Read the model definition and answer for the solid it produces. Units are mm, in the model's axes. A direction names the side the tool comes from. Coordinates: 2 decimals unless noted, no trailing zeros. Write each loop counter-clockwise with the first axis right and the second up, starting at its lowest first coordinate (ties: lowest second). Pieces come first, ordered by that corner, then holes. Notation, with made-up numbers: (-15.75, 18.25) - (-9.75, 18.25) arc R10 ccw to (-9.75, 30.25) - close; hole circle Ø5 at (23.5, 38). An arc over 180 degrees is marked (long way). Use a Markdown table: item, result.
Autodesk Inventor part; units mm, degrees
ref_plane "YZ Plane" through (0, 0, 0) normal (1, 0, 0) x (0, 1, 0)
ref_plane "XZ Plane" through (0, 0, 0) normal (0, 1, 0) x (-1, 0, 0)
ref_plane "XY Plane" through (0, 0, 0) normal (0, 0, 1) x (1, 0, 0)
sketch "Sketch1" plane through (0, 0, 0) normal (0, 1, 0) x (-1, 0, 0)
  line L0 (-40.135, 30.32) -> (40.135, 30.32)
  line L1 (40.135, 30.32) -> (40.135, -30.32)
  line L2 (40.135, -30.32) -> (-40.135, -30.32)
  line L3 (-40.135, -30.32) -> (-40.135, 30.32)
  line L4 (-40.135, 30.32) -> (40.135, -30.32) construction
  line L5 (40.135, 30.32) -> (-40.135, -30.32) construction
  point P0 (0, 0)
  dimension "d0" = 80.27
  dimension "d1" = 60.64
extrude "Extrusion1" add sketch "Sketch1" along normal blind 4.75
sketch "Sketch2" plane through (0, 4.75, 0) normal (0, 1, 0) x (1, 0, 0)
  line L0 (-40.135, -30.32) -> (40.135, -30.32)
  line L1 (40.135, -30.32) -> (40.135, 30.32)
  line L2 (-40.135, -30.32) -> (40.135, -30.32)
  line L3 (40.135, -30.32) -> (40.135, -25.57)
  line L4 (40.135, -25.57) -> (-40.135, -25.57)
  line L5 (-40.135, -25.57) -> (-40.135, -30.32)
  line L6 (-40.135, 30.32) -> (40.135, 30.32)
  line L7 (40.135, 30.32) -> (40.135, 25.57)
  line L8 (40.135, 25.57) -> (-40.135, 25.57)
  line L9 (-40.135, 25.57) -> (-40.135, 30.32)
  line L10 (-40.135, -25.57) -> (-35.385, -25.57)
  line L11 (-35.385, -25.57) -> (-35.385, 25.57)
  line L12 (-35.385, 25.57) -> (-40.135, 25.57)
  line L13 (-40.135, 25.57) -> (-40.135, -25.57)
  line L14 (40.135, 25.57) -> (35.385, 25.57)
  line L15 (35.385, 25.57) -> (35.385, -25.57)
  line L16 (35.385, -25.57) -> (40.135, -25.57)
  line L17 (40.135, -25.57) -> (40.135, 25.57)
  point P0 (0, 0)
  dimension "d4" = 4.75
  dimension "d5" = 4.75
  dimension "d6" = 4.75
  dimension "d7" = 4.75
extrude "Extrusion2" add sketch "Sketch2" along normal blind 50.72 contours L5 L4 L1 L0 | L13 L8 L11 L4 | L4 L15 L8 L1 | L9 L6 L1 L8
sketch "Sketch3" plane through (0, 55.47, 0) normal (0, 1, 0) x (1, 0, 0)
  line L0 (40.135, -30.32) -> (-40.135, -30.32)
  line L1 (-40.135, -30.32) -> (-40.135, 30.32)
  line L2 (-40.135, 30.32) -> (40.135, 30.32)
  line L3 (40.135, 30.32) -> (40.135, -30.32)
  point P0 (0, 0)
extrude "Extrusion3" add sketch "Sketch3" along normal blind 4.75
sketch "Sketch4" plane through (40.135, 0, 30.32) normal (1, 0, 0) x (0, 0, -1)
  line L0 (0, 60.22) -> (60.64, 60.22)
  line L1 (0, 0) -> (0, 60.22)
  line L2 (60.64, 0) -> (60.64, 60.22)
  line L3 (60.64, 0) -> (0, 0)
  point P0 (30.32, 0)
  point P1 (30.32, 30.11)
hole "Hole1" at (40.135, 30.11, 0) direction (-1, 0, 0) diameter 11.4554 end up to surface
sketch "Sketch5" plane through (0, 60.22, 0) normal (0, 1, 0) x (1, 0, 0)
  line L0 (-40.135, -30.32) -> (40.135, -30.32)
  line L1 (40.135, -30.32) -> (40.135, 30.32)
  line L2 (40.135, 30.32) -> (-40.135, 30.32)
  line L3 (-40.135, 30.32) -> (-40.135, -30.32)
  point P0 (0, 0)
  point P1 (-24.635, 0)
  point P2 (15.015, 0)
  dimension "d19" = 15.5
  dimension "d20" = 25.12
hole "Hole2" at (-24.635, 60.22, 0) at (15.015, 60.22, 0) direction (0, -1, 0) diameter 11.4554 end up to surface
properties part number "Reservoir" material "PMMA Plastic"
(1) For faces 1 (the cylindrical face through (-30.314, 57.812, -0.746)), 2 (the flat face through (0, 4.75, 0)), 3 (the cylindrical face through (37.73, 24.43, 0.75)), determine the directions among +Z, -Z, +X, -X, +Y, -Y from which every point of the face is accessible in a straight line to the end or side of a thin tool.
Report:
| item | result |
|---|---|
| face 1 | +Y |
| face 2 | none |
| face 3 | +X |
(2) Straight lines are drawn through the part: L1, parallel to X at y = 59.25, z = 0 (3 decimals); L2, parallel to X at y = 26, z = 11 (3 decimals); L3, parallel to Y at x = -0.5, z = 6.5. For each, find the intervals that lie inside material, in ascending order.
Report:
| item | result |
|---|---|
| L1 | x = -40.135 to -30.363, -18.907 to 9.287, 20.743 to 40.135 |
| L2 | x = -40.135 to -35.385, 35.385 to 40.135 |
| L3 | y = 0 to 4.75, 55.47 to 60.22 |
(3) The mould has two halves that part along Z. Classify faces 4 (the flat face through (-1, 30, -30.32)), 5 (the flat face through (35.385, 24, 0)), 6 (the flat face through (-40.135, 30, 0)): pulls with the +Z half, pulls with the -Z half, needs draft (parallel to the pull), parting line crosses it, or undercut.
Report:
| item | result |
|---|---|
| face 4 | pulls with the -Z half |
| face 5 | undercut |
| face 6 | needs draft |
(4) A cutting plane is placed at D-D, the plane y = 30.11. Write down the section's boundary in (x, z) (3 decimals), and give its area (3 significant figures).
Report:
| item | result |
|---|---|
| outline | (-40.135, -30.32) - (40.135, -30.32) - (40.135, -5.728) - (35.385, -5.728) - (35.385, -25.57) - (-35.385, -25.57) - (-35.385, 25.57) - (35.385, 25.57) - (35.385, 5.728) - (40.135, 5.728) - (40.135, 30.32) - (-40.135, 30.32) - close |
| area | 1,190 mm² |
(5) Each of these flat-tipped pins is pushed along its axis until it touches: P1, Ø7, axis at y = 30.11, z = 0, coming from the +X side (3 decimals); P2, Ø10.5, axis at x = -24.635, z = 0, coming from the +Y side. Where does it stop, or does it pass through?
Report:
| item | result |
|---|---|
| P1 | stops at x = -35.385 |
| P2 | stops at y = 4.75 |
(6) A cutting plane is placed at A-A, the plane y = 54. Write down the section's boundary in (x, z) (3 decimals), and give its area (3 significant figures).
Report:
| item | result |
|---|---|
| outline | (-40.135, -30.32) - (40.135, -30.32) - (40.135, 30.32) - (-40.135, 30.32) - close; hole (-35.385, -25.57) - (35.385, -25.57) - (35.385, 25.57) - (-35.385, 25.57) - close |
| area | 1,250 mm² |
(7) A cutting plane is placed at B-B, the plane z = 11.5. Write down the section's boundary in (x, y) (3 decimals), and give its area (3 significant figures).
Report:
| item | result |
|---|---|
| outline | (-40.135, 0) - (40.135, 0) - (40.135, 60.22) - (-40.135, 60.22) - close; hole (-35.385, 4.75) - (35.385, 4.75) - (35.385, 55.47) - (-35.385, 55.47) - close |
| area | 1,240 mm² |
(8) A cutting plane is placed at C-C, the plane z = 0. Write down the section's boundary in (x, y) (3 decimals), and give its area (3 significant figures).
Report:
| item | result |
|---|---|
| outline | (-40.135, 0) - (40.135, 0) - (40.135, 24.382) - (35.385, 24.382) - (35.385, 4.75) - (-35.385, 4.75) - (-35.385, 55.47) - (-30.363, 55.47) - (-30.363, 60.22) - (-40.135, 60.22) - close; (-18.907, 55.47) - (9.287, 55.47) - (9.287, 60.22) - (-18.907, 60.22) - close; (20.743, 55.47) - (35.385, 55.47) - (35.385, 35.838) - (40.135, 35.838) - (40.135, 60.22) - (20.743, 60.22) - close |
| area | 1,080 mm² |
